from build123d import *

# Parameters (mm, degrees)
F1_R     = 8.89
F1_R_2   = 5.969
F3_DEPTH = 3.556
F5_R     = 8.89
F5_R_2   = 7.62
F7_DEPTH = 3.556


# Not quite as in the source:
# - a feature of the source that left no trace in its solid (it failed there, or was rolled back) is left out
# - a pattern or mirror of a feature is missing from the dataset's text; its kind, count and spacing are read off the source's solid


with BuildPart() as f2:
    # F2: sweep along a path in F0
    with BuildLine(Plane.XY) as f2_path:
        Line((0, 0), (0, 70.4088))
        ThreePointArc((0, 70.4088), (13.97, 84.3788), (27.94, 70.4088))
        Line((27.94, 70.4088), (27.94, 0))
        Line((27.94, 0), (27.94, -3.556))
    # F1 (on Front) → F2 (sweep)
    with BuildSketch(Plane.XZ):
        Circle(F1_R)
        Circle(F1_R_2, mode=Mode.SUBTRACT)
    sweep(path=f2_path.line)

    # F3 (add): a face of the model
    f3_faces = [f2.faces().sort_by_distance(p)[0] for p in [
        (-8.6385528286, 0, 0),
    ]]
    extrude(f3_faces, amount=F3_DEPTH)

    # F5 (on face) → F7 (cut)
    with BuildSketch(Plane.XZ.offset(3.556)):
        with Locations((27.94, 0)):
            Circle(F5_R)
        with Locations((27.94, 0)):
            Circle(F5_R_2, mode=Mode.SUBTRACT)
    f7 = extrude(amount=-F7_DEPTH, mode=Mode.SUBTRACT)

    # F7_copies: F7 across plane
    add(f7.mirror(Plane(origin=(13.97, 0, 0), x_dir=(0, 0, -1), z_dir=(-1, 0, 0))), mode=Mode.SUBTRACT)


solid = f2.part
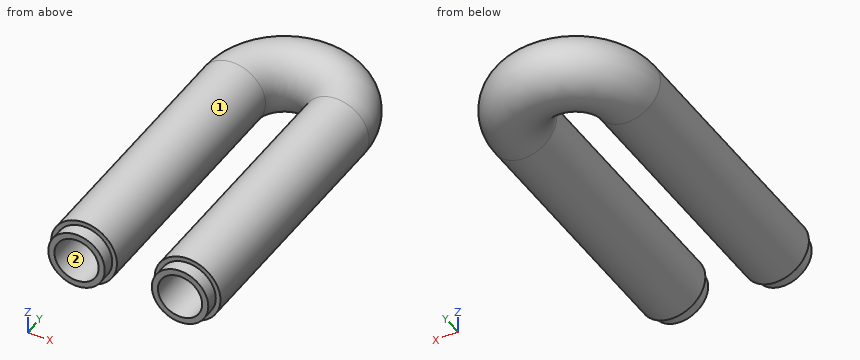
Could you check a few things on this model? Use its own coordinates, in mm. Face numbers are marked on the shaded views. Give positions to 0.01 mm unless a question says otherwise; leave off trailing zeros. Order: outer loops, then holes, each group sorted by start corner. A loop starts at its lowest first (then second) coordinate and runs counter-clockwise, first axis right, second up.
Item 1: If we section it at C-C, the plane y = 77: Count the separate pieces of the cut face and the enclosed holes in it, plus the area to 3 significant figures.
Item 2: If we section it at A-A, the plane z = 0: Write out the boundary of the cut face in (x, y).
Item 3: I need wall thicknesses on line 1 (X direction, y = 48.5, z = 0); line 2 (Z direction, x = 0, y = 50.5); line 3 (Y direction, x = 8, z = -2). Which ranges of each line are inside material? Lowest first, please.
Item 4: If we section it at B-B, the plane y = 59.5: Write out the boundary of the cut face in (x, z).
Item 5: I'm going to push flat-ended pins straight in: pin 1 (4 mm diameter, centred on y = 61, z = -2.5, fed in from +X); pin 2 (2 mm diameter, centred on y = 62, z = -6.5, fed in from -X); pin 3 (8 mm diameter, centred on x = 14, z = -5, fed in from -Y). Where does each tip first touch, or does it pass through?
Item 6: If we mould it in two halves opening along Z, with no side actions, what happens to the marked faces 1 and 2? For each: pulls with the +Z half, pulls with the -Z half, needs draft (parallel to the pull), parting line crosses it, or undercut.
Values:
1. separate pieces: 1
1. enclosed holes: 2
1. area: 358 mm2
2. outline: (-8.89, 0) - (-7.62, 0) - (-7.62, -3.56) - (-5.97, -3.56) - (-5.97, 70.41) arc R19.94 cw to (33.91, 70.41) - (33.91, -3.56) - (35.56, -3.56) - (35.56, 0) - (36.83, 0) - (36.83, 70.41) arc R22.86 ccw to (-8.89, 70.41) - close; (5.97, -3.56) - (7.62, -3.56) - (7.62, 0) - (8.89, 0) - (8.89, 70.41) arc R5.08 cw to (19.05, 70.41) - (19.05, 0) - (20.32, 0) - (20.32, -3.56) - (21.97, -3.56) - (21.97, 70.41) arc R8 ccw to (5.97, 70.41) - close
3. line 1: x = -8.89 to -5.97, 5.97 to 8.89, 19.05 to 21.97, 33.91 to 36.83
3. line 2: z = -8.89 to -5.97, 5.97 to 8.89
3. line 3: y = 0 to 76.24, 89.07 to 92.24
4. outline: circle Ø17.78 at (0, 0); circle Ø17.78 at (27.94, 0); hole circle Ø11.94 at (0, 0); hole circle Ø11.94 at (27.94, 0)
5. pin 1: stops at x = 36.82
5. pin 2: stops at x = -6.98
5. pin 3: stops at y = 74.79
6. face 1: parting line crosses it
6. face 2: undercut
